```python
from build123d import *

# Parameters (mm, degrees)
F0_R         = 50.8
F1_DEPTH     = 31.75
F2_R         = 5.08
F3_R         = 9.525
F4_DEPTH     = 31.751
F1_FACE_R    = 45.72
F1_FACE_R_2  = 9.525
F5_DEPTH     = 6.35
F1_FACE1_R   = 45.72
F1_FACE1_R_2 = 9.525
F6_DEPTH     = 6.35
F7_R         = 19.05
F7_R_2       = 9.525
F8_DEPTH     = 76.2
F10_R        = 19.05
F11_DEPTH    = 76.2


with BuildPart() as f1:
    # F0 (on Front) → F1 (new body)
    with BuildSketch(Plane.XZ):
        Circle(F0_R)
    extrude(amount=F1_DEPTH)

    # F2
    f2_edges = [f1.edges().sort_by_distance(p)[0] for p in [
        (-50.8, -31.75, 0),
        (-50.8, 0, 0),
    ]]
    fillet(f2_edges, radius=F2_R)

    # F3 (on face) → F4 (cut, through all)
    with BuildSketch(Plane.XZ.offset(31.75)):
        Circle(F3_R)
    extrude(amount=-F4_DEPTH, mode=Mode.SUBTRACT)

    # F1_face (on face) → F5 (cut)
    with BuildSketch(Plane.XZ.offset(31.75)):
        Circle(F1_FACE_R)
        Circle(F1_FACE_R_2, mode=Mode.SUBTRACT)
    extrude(amount=-F5_DEPTH, mode=Mode.SUBTRACT)

    # F1_face1 (on face) → F6 (cut)
    with BuildSketch(Plane(origin=(0, 0, 0), x_dir=(1, 0, 0), z_dir=(0, 1, 0))):
        Circle(F1_FACE1_R)
        Circle(F1_FACE1_R_2, mode=Mode.SUBTRACT)
    extrude(amount=-F6_DEPTH, mode=Mode.SUBTRACT)

    # F7 (on face) → F8 (join)
    with BuildSketch(Plane.XZ.offset(25.4)):
        Circle(F7_R)
        Circle(F7_R_2, mode=Mode.SUBTRACT)
    extrude(amount=F8_DEPTH)

    # F9: F1 across plane


with BuildPart() as f1_1:
    add(f1.part)
    add(f1.part.mirror(Plane.YZ))

    # F10 (on face) → F11 (join)
    with BuildSketch(Plane(origin=(0, -6.35, 0), x_dir=(-1, 0, 0), z_dir=(0, 1, 0))):
        Circle(F10_R)
        with BuildLine():
            ThreePointArc((-9.525, 0), (0, 9.525), (9.525, 0))
            ThreePointArc((9.525, 0), (0, -9.525), (-9.525, 0))
        make_face(mode=Mode.SUBTRACT)
    extrude(amount=F11_DEPTH)


solid = f1_1.part
```
The listing builds one solid part. Answer for the finished solid, in the listing's coordinates (mm). A direction names the side the tool comes from. Give positions to 0.01 mm unless a question says otherwise; leave off trailing zeros. Loops run counter-clockwise (first coordinate to the right, second up) from the corner with the lowest first, then second, coordinate; pieces in that order, holes last. Notation, with made-up numbers: M 1,-14.5 L 10,-14.5 A37 cw 10,21.5 Z; hole C 15.25,68.25 d2. An arc over 180 degrees is marked long. One line per item, written item: value.
1. Each of these flat-tipped pins is pushed along its axis until it touches: P1, Ø6, axis at x = 9, y = -71, coming from the +Z side; P2, Ø8, axis at x = -32, y = -33.5, coming from the -Z side; P3, Ø12, axis at x = 22.5, y = -72.5, coming from the +Z side. Where does it stop, or does it pass through?
Found:
P1: z = 18.08
P2: z = -39.41
P3: z = 9.52
2. Section B-B on y = 24.5 is taken. Determine the outline of the cut face in (x, z) (3 decimals), plus the area to 3 significant figures.
Found:
outline: C 0,0 d38.1; hole C 0,0 d19.05
area: 855 mm^2
3. Find the intervals of material crossed by probe 1 along Z at (x, y) = (0, -4.5) (3 decimals); probe 2 along Z at (x, y) = (0, -3) (3 decimals); probe 3 along Y at (x, z) = (-44.5, -1.5), in increasing order.
Found:
probe 1: -50.767 to -45.72, -19.05 to -9.525, 9.525 to 19.05, 45.72 to 50.767
probe 2: -50.355 to -45.72, -19.05 to -9.525, 9.525 to 19.05, 45.72 to 50.355
probe 3: -25.4 to -6.35
4. Section C-C on y = -19.5 is taken. Determine the outline of the cut face in (x, z) (3 decimals).
Found:
outline: C 0,0 d101.6; hole C 0,0 d19.05
5. For faces 3 (the face through (-1, -25.4, -20)), 4 (the face through (4, -101.6, 9)), 5 (the face through (43.61, -3.13, -13.73)), determine the directions among +Z, -Z, +X, -X, +Y, -Y from which every point of the face is accessible in a straight line to the end or side of a thin tool.
Found:
face 3: -Y
face 4: +Z, -Z, +X, -X, -Y
face 5: +Y
6. Section A-A on x = 0 is taken. Determine the outline of the cut face in (y, z) (3 decimals), plus the area to 3 significant figures.
Found:
outline: M -101.6,-19.05 L -25.4,-19.05 L -25.4,-45.72 L -31.75,-45.72 A5.08 ccw -26.67,-50.8 L -5.08,-50.8 A5.08 ccw 0,-45.72 L -6.35,-45.72 L -6.35,-19.05 L 69.85,-19.05 L 69.85,-9.525 L -101.6,-9.525 Z; M -101.6,9.525 L 69.85,9.525 L 69.85,19.05 L -6.35,19.05 L -6.35,45.72 L 0,45.72 A5.08 ccw -5.08,50.8 L -26.67,50.8 A5.08 ccw -31.75,45.72 L -25.4,45.72 L -25.4,19.05 L -101.6,19.05 Z
area: 4,580 mm^2
7. For a pull along X with two mould halves and no side action, classify faces 1 (the face through (43.61, -28.62, 13.73)), 2 (the face through (-4, 69.85, 9)) as pulls with the +X half, pulls with the -X half, needs draft (parallel to the pull), parting line crosses it, or undercut.
Found:
face 1: undercut
face 2: needs draft
